Autodesk Inventor part; units mm, degrees
ref_plane "YZ Plane" through (0, 0, 0) normal (1, 0, 0) x (0, 1, 0)
ref_plane "XZ Plane" through (0, 0, 0) normal (0, 1, 0) x (-1, 0, 0)
ref_plane "XY Plane" through (0, 0, 0) normal (0, 0, 1) x (1, 0, 0)
sketch "Sketch1" plane through (0, 0, 0) normal (0, 1, 0) x (-1, 0, 0)
  line L0 (25, -25) -> (-25, -25)
  line L1 (-25, -25) -> (-25, 25)
  line L2 (-25, 25) -> (25, 25)
  line L3 (25, 25) -> (25, -25)
  line L4 (-20, -20) -> (20, -20)
  line L5 (20, -20) -> (20, 20)
  line L6 (20, 20) -> (-20, 20)
  line L7 (-20, 20) -> (-20, -20)
  point P0 (0, 0)
  dimension "d0" = 50
  dimension "d1" = 50
  dimension "d2" = 25
  dimension "d3" = 25
  dimension "d4" = 5
extrude "Extrusion1" add sketch "Sketch1" along normal blind 539
fillet "Fillet1" radius 2 4 edges at (25, 269.5, -25) (25, 269.5, 25) (-25, 269.5, 25) (-25, 269.5, -25)
sketch "Sketch2" plane through (-23, 0, 25) normal (0, 0, 1) x (1, 0, 0)
  line L0 (-78.8613, 79.786) -> (128.2392, 79.786)
  line L1 (0, 539) -> (46, 539)
  line L2 (48, 0) -> (48, 539)
  point P0 (23, 0)
  point P1 (30.5, 145.786)
  point P2 (30.5, 13.786)
  dimension "d19" = 459.214
  dimension "d22" = 66
  dimension "d23" = 66
  dimension "d24" = 17.5
  dimension "d25" = 0
hole "Hole1" at (7.5, 145.786, 25) at (7.5, 13.786, 25) direction (0, 0, -1) diameter 8 end through all
equation "\"d0\" = w"
equation "\"d1\" = d0"
equation "\"d4\" = t"
equation "\"d5\" = L"
equation "\"w\" = support_frame_squareBarDimension"
equation "\"t\" = support_frame_squareBarThickness"
equation "\"L\" = 539"
equation "\"hoop_angle_z\" = 45deg"
equation "\"hoop_bearing_length\" = 5deg"
equation "\"hoop_bushing12_od\" = -2 * hoop_thickness_large + hoop_width_large + hoop_bushing12_radialInterference"
equation "\"hoop_bushing12_radialInterference\" = 0"
equation "\"hoop_bushing12_thickness\" = -hoop_width_medium + hoop_bushing12_od - 2 * hoop_bushing12_radialInterference"
equation "\"hoop_bushing23_od\" = -2 * hoop_thickness_medium + hoop_width_medium + hoop_bushing23_radialInterference"
equation "\"hoop_bushing23_radialInterference\" = 0"
equation "\"hoop_bushing23_thickness\" = -hoop_width_small + hoop_bushing23_od - 2 * hoop_bushing23_radialInterference"
equation "\"hoop_cable_diam\" = 5"
equation "\"hoop_cable_pulley_diam\" = 22"
equation "\"hoop_tabs_hole\" = 12"
equation "\"hoop_tabs_thickness\" = 6"
equation "\"hoop_thickness_large\" = 4"
equation "\"hoop_thickness_medium\" = 3.2"
equation "\"hoop_thickness_small\" = 2"
equation "\"hoop_width_large\" = 51"
equation "\"hoop_width_medium\" = 33.7"
equation "\"hoop_width_small\" = 25.4"
equation "\"rack_tooth_addendum\" = 5"
equation "\"rack_tooth_dedendum\" = 5"
equation "\"rack_tooth_thickness\" = 5"
equation "\"secure_arm_angle\" = 35deg"
equation "\"secure_arm_radii\" = 9"
equation "\"sm_varx_member_tolerance\" = 0"
equation "\"sm_varx_pinPlate_holeDiameter\" = 5"
equation "\"sm_varx_pinPlate_thickness\" = 5"
equation "\"sm_varx_squareBarThickness\" = 2.5"
equation "\"support_baseClamp_platformLengthBuffer\" = 35"
equation "\"support_baseClamp_platformThickness\" = 15"
equation "\"support_baseClamp_platformWidthBuffer\" = 0"
equation "\"support_baseClamp_sleeveHoleDiameter\" = 12"
equation "\"support_baseClamp_sleeveSweepTerminationAngle\" = 55deg"
equation "\"support_baseClamp_thickness\" = 8"
equation "\"support_frame_endHoleBuffer\" = 45"
equation "\"support_frame_squareBarFillet\" = 2"
equation "\"support_frame_squareBarThickness\" = 5"
equation "\"wheelchair_deployed_height\" = 914"
equation "\"wheelchair_deployed_length\" = 1067"
equation "\"wheelchair_deployed_width\" = 635"
equation "\"wheelchatir_pos_deploy_angle_0\" = 65deg"
equation "\"wheelchatir_pos_store_angle_0\" = 90deg"
equation "\"wheelchatir_pos_deploy_angle_1\" = 20deg"
equation "\"wheelchatir_pos_store_angle_1\" = 20deg"
properties part number "support_frame_z" material "Steel, Mild"
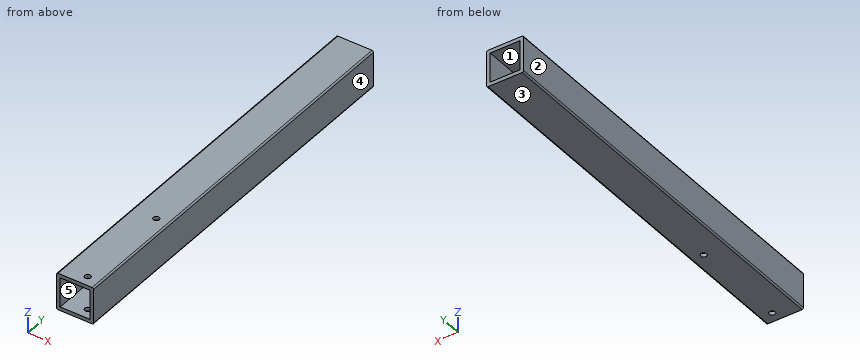
Geometry: final body of the model. Coordinates: model frame, mm. Face numbers are marked on the shaded views. A direction names the side the tool comes from. Round coordinates to 2 decimals unless told otherwise and drop trailing zeros. Order: outer loops, then holes, each group sorted by start corner. A loop starts at its lowest first (then second) coordinate and runs counter-clockwise, first axis right, second up. Notation, with made-up numbers: (60.5, 38) -> (66.5, 38) arc R26 ccw to (66.5, 69) -> close; hole circle Ø10 at (18, 3). An arc over 180 degrees is marked (long way). Write each question's results on one line, items separated by ' | '.
Q1. Ray query, line 1 along Y through (x, z) = (7.5, 22.45); line 2 along Z through (x, y) = (-17, 413). Return the intervals inside material, ascending.
Response values:
line 1: 0 to 9.79, 17.79 to 141.79, 149.79 to 539 | line 2: -25 to -20, 20 to 25
Q2. Section query A-A (z = 14). Output: boundary loops of the cut face in (x, y).
Response values:
outline: (-25, 0) -> (-20, 0) -> (-20, 539) -> (-25, 539) -> close; (20, 0) -> (25, 0) -> (25, 539) -> (20, 539) -> close
Q3. Section query B-B (y = 77). Output: boundary loops of the cut face in (x, z), and give its area (3 significant figures).
Response values:
outline: (-25, -23) arc R2 ccw to (-23, -25) -> (23, -25) arc R2 ccw to (25, -23) -> (25, 23) arc R2 ccw to (23, 25) -> (-23, 25) arc R2 ccw to (-25, 23) -> close; hole (-20, -20) -> (20, -20) -> (20, 20) -> (-20, 20) -> close | area: 897 mm²
Q4. Access query for the marked faces 4 and 5. Directions: +Z, -Z, +X, -X, +Y, -Y. A direction counts if a zero-diameter tool reaches every point of the face in a straight line with its end or side. Return the directions, or none.
Response values:
face 4: +Z, -Z, +X, +Y, -Y | face 5: +Y, -Y
Q5. Pull-direction query (Z, two-part tool) for the marked faces 1, 2 and 3; classes: released by +Z, released by -Z, zero draft, split by the parting line, or undercut.
Response values:
face 1: undercut | face 2: zero draft | face 3: released by -Z
